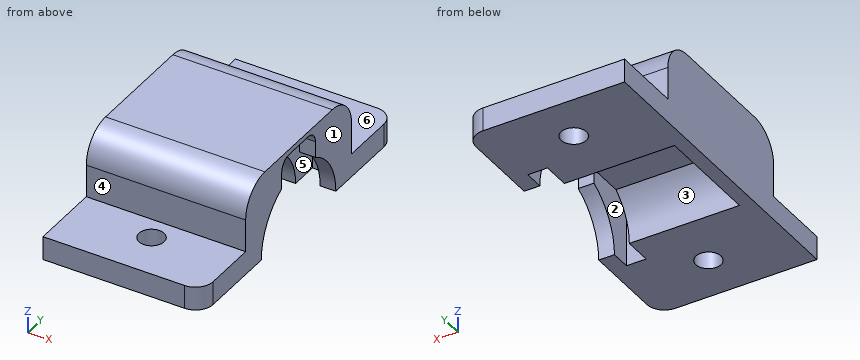
from build123d import *

# Parameters (mm, degrees)
SKETCH1_W           = 20.25
SKETCH1_H           = 40
BODY_DEPTH          = 3
SKETCH2_W           = 20.25
SKETCH2_H           = 22
HIROSE_DEPTH        = 8.15
SKETCH3_W           = 2
SKETCH3_H           = 7.75
SKETCH4_W           = 2.5
SKETCH4_H           = 20.5
HIROSE_MID_DEPTH    = 10.4
CUT_EXTRUDE2_DEPTH  = 2
FILLET1_R           = 1.5
SKETCH7_W           = 14
SKETCH7_H           = 6.75
BOSS_EXTRUDE3_START = 14
BOSS_EXTRUDE3_DEPTH = 14
FILLET2_R           = 3
FILLET3_R           = 4
SKETCH9_R           = 1.6
CUT_EXTRUDE3_DEPTH  = 46.568464973
FILLET4_R           = 2.25


with BuildPart() as part:
    # Sketch1 → body (new body)
    with BuildSketch(Plane.XY):
        with Locations((10.125, 20)):
            Rectangle(SKETCH1_W, SKETCH1_H)
    extrude(amount=BODY_DEPTH)

    # Sketch2 → hirose (add)
    with BuildSketch(Plane.XY.offset(3)):
        with Locations((10.125, 20)):
            Rectangle(SKETCH2_W, SKETCH2_H)
    extrude(amount=HIROSE_DEPTH)

    # Sketch3 → hirose-front (revolve, cut)
    with BuildSketch(Plane(origin=(0, 0, 0), x_dir=(-1, 0, 0), z_dir=(0, 0, -1))):
        with Locations((-19.25, 23.875)):
            Rectangle(SKETCH3_W, SKETCH3_H)
    revolve(axis=Axis((20.25, 20, 0), (-1, 0, 0)), mode=Mode.SUBTRACT)

    # Sketch4 → hirose-mid (cut)
    with BuildSketch(Plane(origin=(0, 0, 0), x_dir=(-1, 0, 0), z_dir=(0, 0, -1))):
        with Locations((-17, 20)):
            Rectangle(SKETCH4_W, SKETCH4_H)
    extrude(amount=-HIROSE_MID_DEPTH, mode=Mode.SUBTRACT)

    # Sketch5 → Cut-Extrude2 (cut)
    with BuildSketch(Plane(origin=(20.25, 0, 0), x_dir=(0, 0, -1), z_dir=(1, 0, 0))):
        with BuildLine():
            Line((-10.5, 16.5), (-10.5, 23.5))
            Line((-10.5, 23.5), (-6.914658343, 23.5))
            ThreePointArc((-6.914658343, 23.5), (-7.75, 20), (-6.914658343, 16.5))
            Line((-6.914658343, 16.5), (-10.5, 16.5))
        make_face()
    extrude(amount=-CUT_EXTRUDE2_DEPTH, mode=Mode.SUBTRACT)

    # Fillet1
    # the kernel refuses this fillet: 1.5 mm, written as the material it adds along each edge
    with BuildSketch(Plane(origin=(20.25, 23.5, 10.5), x_dir=(0, -1, 0), z_dir=(-1, 0, 0)), Plane(origin=(20.25, 16.5, 10.5), x_dir=(0, 0, -1), z_dir=(-1, 0, 0))) as fillet1_piece_1:
        with BuildLine():
            CenterArc((FILLET1_R, -FILLET1_R), FILLET1_R, 90, 90)
            Line((0, -FILLET1_R), (0, 0))
            Line((0, 0), (FILLET1_R, 0))
        make_face()
    extrude(amount=2)

    # Sketch7 → Cut-Revolve2 (revolve, cut)
    with BuildSketch(Plane(origin=(0, 0, 0), x_dir=(-1, 0, 0), z_dir=(0, 0, -1))):
        with Locations((-8.75, 23.375)):
            Rectangle(SKETCH7_W, SKETCH7_H)
    revolve(axis=Axis((15.75, 20, 0), (-1, 0, 0)), mode=Mode.SUBTRACT)

    # Sketch8 → Boss-Extrude3 (add)
    with BuildSketch(Plane(origin=(1.75, 0, 0), x_dir=(0, 0, -1), z_dir=(1, 0, 0)).offset(BOSS_EXTRUDE3_START)):
        with BuildLine():
            Line((-5.45, 23.98246155), (-5.45, 16.01753845))
            ThreePointArc((-5.45, 16.01753845), (-6.75, 20), (-5.45, 23.98246155))
        make_face()
    extrude(amount=-BOSS_EXTRUDE3_DEPTH)

    # Fillet2
    fillet2_edges = [part.edges().sort_by_distance(p)[0] for p in [
        (17, 9.75, 10.4),
        (17, 30.25, 10.4),
    ]]
    fillet(fillet2_edges, radius=FILLET2_R)

    # Fillet3
    fillet3_edges = [part.edges().sort_by_distance(p)[0] for p in [
        (10.125, 9, 11.15),
        (10.125, 31, 11.15),
    ]]
    fillet(fillet3_edges, radius=FILLET3_R)

    # Sketch9 → Cut-Extrude3 (cut, through all)
    with BuildSketch(Plane.XY.offset(3)):
        with Locations((10.125, 34)):
            Circle(SKETCH9_R)
        with Locations((10.125, 6)):
            Circle(SKETCH9_R)
    extrude(amount=-CUT_EXTRUDE3_DEPTH, mode=Mode.SUBTRACT)

    # Fillet4
    fillet4_edges = [part.edges().sort_by_distance(p)[0] for p in [
        (20.25, 40, 1.5),
        (20.25, 0, 1.5),
    ]]
    fillet(fillet4_edges, radius=FILLET4_R)


solid = part.part
CAD build for the part. Positions are in the model's coordinates, mm. Face numbers are marked on the shaded views. A direction names the side the tool comes from. Give positions to 0.01 mm unless a question says otherwise; leave off trailing zeros. Loops run counter-clockwise (first coordinate to the right, second up) from the corner with the lowest first, then second, coordinate; pieces in that order, holes last. Notation, with made-up numbers: M -38,-0.5 L -17,-0.5 A28 ccw -17,38.5 Z; hole C -9,65.25 d4. An arc over 180 degrees is marked long. Answer in a Markdown table with one row per item. Add a question column.
Item 1: Mould opens along X. For the marked faces 1, 2 and 3 say: +X half, -X half, draft (parallel to the pull), parting line (faces both ways), or undercut.
Item 2: Band-saw the part on B-B on x = 16.5. Give the cut face in (y, z).
Item 3: Band-saw the part on D-D on z = 1.5. Give the cut face in (x, y) (3 decimals), then the cut area to 3 significant figures.
Item 4: Probe probe 1 along X at (y, z) = (10, 7.75); probe 2 along Y at (x, z) = (16.5, 6); probe 3 along Z at (x, y) = (6.75, 17). List the from-to ranges inside material, lowest first.
Item 5: Drop flat-ended pins along their axis: P1, Ø6, axis at x = 12, z = 5.5, coming from the +Y side; P2, Ø0.6, axis at x = 19, z = 7.5, coming from the +Y side; P3, Ø4.5, axis at y = 19.5, z = 3.5, coming from the +X side; P4, Ø2, axis at x = 6.5, z = 5, coming from the -Y side. Give the stop position or say it passes through.
Item 6: Band-saw the part on C-C on y = 21. Give the cut face in (x, z), then the cut area to 3 significant figures.
Item 7: Band-saw the part on A-A on y = 6. Give the cut face in (x, z) (3 decimals), then the cut area to 4 significant figures.
Item 8: Tool access for the marked faces 4, 5 and 6: list every direction of +Z, -Z, +X, -X, +Y, -Y with a clear straight run to the whole face (end or side of a thin tool).
Reply:
| question | item | result |
|---|---|---|
| 1 | face 1 | +X half |
| 1 | face 2 | undercut |
| 1 | face 3 | draft |
| 2 | outline | M 0,0 L 9.75,0 L 9.75,7.4 A3 cw 12.75,10.4 L 27.25,10.4 A3 cw 30.25,7.4 L 30.25,0 L 40,0 L 40,3 L 31,3 L 31,7.15 A4 ccw 27,11.15 L 13,11.15 A4 ccw 9,7.15 L 9,3 L 0,3 Z |
| 3 | outline | M 0,0 L 18,0 A2.25 ccw 20.25,2.25 L 20.25,12.397 L 18.25,12.397 L 18.25,9.75 L 15.75,9.75 L 15.75,13.419 L 1.75,13.419 L 1.75,26.581 L 15.75,26.581 L 15.75,30.25 L 18.25,30.25 L 18.25,27.603 L 20.25,27.603 L 20.25,37.75 A2.25 ccw 18,40 L 0,40 Z; hole C 10.125,6 d3.2; hole C 10.125,34 d3.2 |
| 3 | area | 526 mm^2 |
| 4 | probe 1 | x = 0 to 15.75, 18.25 to 20.25 |
| 4 | probe 2 | y = 9 to 9.75, 30.25 to 31 |
| 4 | probe 3 | z = 5.45 to 11.15 |
| 5 | P1 | stops at y = 40 |
| 5 | P2 | stops at y = 31 |
| 5 | P3 | stops at x = 15.75 |
| 5 | P4 | stops at y = 9 |
| 6 | outline | M 0,0 L 1.75,0 L 1.75,5.45 L 15.75,5.45 L 15.75,10.4 L 18.25,10.4 L 18.25,10.5 L 20.25,10.5 L 20.25,11.15 L 0,11.15 Z |
| 6 | area | 102 mm^2 |
| 7 | outline | M 0,0 L 8.525,0 L 8.525,3 L 0,3 Z; M 11.725,0 L 20.25,0 L 20.25,3 L 11.725,3 Z |
| 7 | area | 51.15 mm^2 |
| 8 | face 4 | +Z, +X, -X, -Y |
| 8 | face 5 | -Z |
| 8 | face 6 | +Z, +X, -X, +Y |
